Source: CAD feature listing. Evaluate the final solid. Frame: model axes, mm. A direction names the side the tool comes from. Give positions to 0.01 mm unless a question says otherwise; leave off trailing zeros. Loops run counter-clockwise (first coordinate to the right, second up) from the corner with the lowest first, then second, coordinate; pieces in that order, holes last. Notation, with made-up numbers: M 15.25,-29 L 51.25,-29 A36 cw 51.25,9 Z; hole C 26,58.5 d6. An arc over 180 degrees is marked long. Answer in a Markdown table with one row per item.
```python
from build123d import *

# Parameters (mm, degrees)
SKETCH1_W           = 27.3
SKETCH1_H           = 27.3
BOSS_EXTRUDE1_DEPTH = 2.2
SKETCH2_W           = 10
SKETCH2_H           = 3.982118458
BOSS_EXTRUDE3_DEPTH = 2


with BuildPart() as part:
    # Sketch1 → Boss-Extrude1 (new body)
    with BuildSketch(Plane(origin=(0, 0, 0), x_dir=(1, 0, 0), z_dir=(0, 1, 0))):
        Rectangle(SKETCH1_W, SKETCH1_H)
    extrude(amount=BOSS_EXTRUDE1_DEPTH)

    # Sketch2 → Boss-Extrude3 (add)
    with BuildSketch(Plane(origin=(0, 2.2, 0), x_dir=(1, 0, 0), z_dir=(0, 1, 0))):
        with Locations((0, 10.141059229)):
            Rectangle(SKETCH2_W, SKETCH2_H)
        Polygon((-12.5, 8.15), (-12.5, -8.85), (12.5, -8.85), (12.5, 8.15), (5, 8.15), (5, 4.167881542), (-5, 4.167881542), (-5, 8.15), align=None)
        with Locations((0, 6.158940771)):
            Rectangle(SKETCH2_W, SKETCH2_H)
    extrude(amount=BOSS_EXTRUDE3_DEPTH)


solid = part.part
```
Q1. Reachability of faces 1 (the flat face through (-9, 3, -8.15)), 2 (the flat face through (0, 3, -12.132)), 3 (the flat face through (9, 3, -8.15)), 4 (the flat face through (-12.5, 3, 0)) from +Z, -Z, +X, -X, +Y, -Y: full face, straight path, thin tool, end or side. Return the list, or none.
Values follow:
| item | result |
|---|---|
| face 1 | -Z, -X, +Y |
| face 2 | -Z, +X, -X, +Y |
| face 3 | -Z, +X, +Y |
| face 4 | +Z, -Z, -X, +Y |
Q2. Section query A-A (z = 0.75). Output: boundary loops of the cut face in (x, y).
Values follow:
| item | result |
|---|---|
| outline | M -13.65,0 L 13.65,0 L 13.65,2.2 L 12.5,2.2 L 12.5,4.2 L -12.5,4.2 L -12.5,2.2 L -13.65,2.2 Z |
Q3. Ray query, probe 1 along Y at (x, z) = (10, -11); probe 2 along Z at (x, y) = (9.5, 2.6); probe 3 along X at (y, z) = (2.5, -1.75). Return the intervals inside material, ascending. Write a range as from..to.
Values follow:
| item | result |
|---|---|
| probe 1 | 0..2.2 |
| probe 2 | -8.15..8.85 |
| probe 3 | -12.5..12.5 |
Q4. Section query B-B (x = -3.5). Output: boundary loops of the cut face in (y, z).
Values follow:
| item | result |
|---|---|
| outline | M 0,-13.65 L 2.2,-13.65 L 2.2,-12.13 L 4.2,-12.13 L 4.2,8.85 L 2.2,8.85 L 2.2,13.65 L 0,13.65 Z |
Q5. Contact query for flat-ended pins moving along their axis: pin 1 Ø0.6 at (y, z) = (3.5, -10.5) entering from -X; pin 2 Ø0.6 at (x, y) = (-9, 3) entering from -Z; pin 3 Ø0.6 at (x, y) = (-1.5, 3.5) entering from +Z. Output: stop coordinate, or through.
Values follow:
| item | result |
|---|---|
| pin 1 | x = -5 |
| pin 2 | z = -8.15 |
| pin 3 | z = 8.85 |
